Design review of the part shown in the three views and the two pictorial views. Dimensions are in mm from the part's minimum x, y and z. A direction names the side the tool comes from. Coordinates: 2 decimals unless noted, no trailing zeros. Loops run counter-clockwise (first coordinate to the right, second up) from the corner with the lowest first, then second, coordinate; pieces in that order, holes last.
Q1. Add section A-A on y = 5. Give the boundary of the cut face in (x, z).
Q2. Machinability: for the marked faces 1 and 2, which of the approach directions +Z, -Z, +X, -X, +Y, -Y give a long, thin tool a straight path to every point of the face, cutting with its end or side? Answer none if there is none.
Q3. Add section B-B on x = 14. Give the boundary of the cut face in (y, z).
Q4. Wall thickness on probe 1 along X at (y, z) = (5, 60); probe 2 along Z at (x, y) = (63, 43.5): over which ranges is each line inside the solid? List them lowest first.
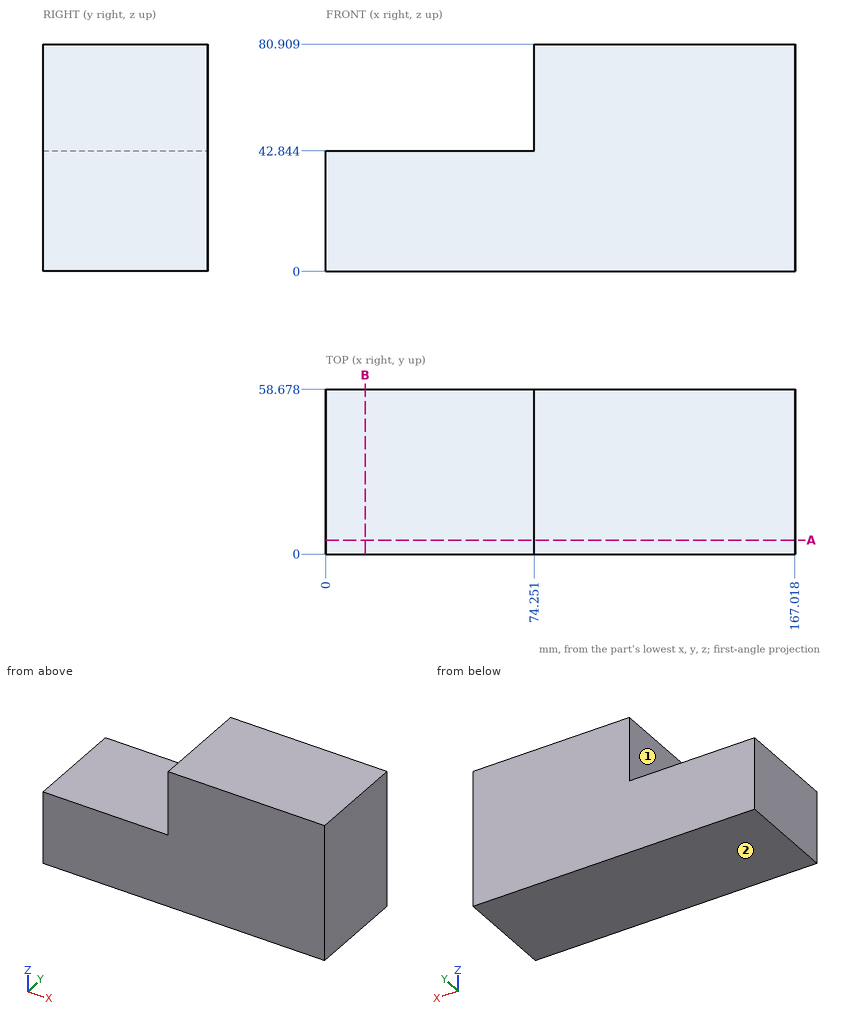
Entries:
1. outline: (0, 0) - (167.02, 0) - (167.02, 80.91) - (74.25, 80.91) - (74.25, 42.84) - (0, 42.84) - close
2. face 1: +Z, -X, +Y, -Y
2. face 2: -Z, +X, -X, +Y, -Y
3. outline: (0, 0) - (58.68, 0) - (58.68, 42.84) - (0, 42.84) - close
4. probe 1: x = 74.25 to 167.02
4. probe 2: z = 0 to 42.84
